Source: CAD feature listing. Evaluate the final solid. Frame: model axes, mm. Round coordinates to 2 decimals unless told otherwise and drop trailing zeros. Write each loop counter-clockwise with the first axis right and the second up, starting at its lowest first coordinate (ties: lowest second). Pieces come first, ordered by that corner, then holes. Notation, with made-up numbers: M -2,3.5 L 52,3.5 A27 cw 52,29.5 Z; hole C 23,36 d3. An arc over 180 degrees is marked long. Answer in a Markdown table with one row per item.
from build123d import *

# Parameters (mm, degrees)
F1_DEPTH = 3.5
F2_R     = 1.8
F3_DEPTH = 8
F4_R     = 1.8
F5_DEPTH = 8


with BuildPart() as f1:
    # F0 (on Top) → F1 (new body, symmetric)
    with BuildSketch(Plane.XY):
        with BuildLine():
            ThreePointArc((30, 1.5), (25.313708, 12.813708), (14, 17.5))
            Line((14, 17.5), (-14, 17.5))
            ThreePointArc((-14, 17.5), (-25.313708, 12.813708), (-30, 1.5))
            Line((-30, 1.5), (-30, -1.5))
            ThreePointArc((-30, -1.5), (-25.313708, -12.813708), (-14, -17.5))
            Line((-14, -17.5), (14, -17.5))
            ThreePointArc((14, -17.5), (25.313708, -12.813708), (30, -1.5))
            Line((30, -1.5), (30, 1.5))
        make_face()
    extrude(amount=F1_DEPTH, both=True)

    # F2 (on face) → F3 (cut)
    with BuildSketch(Plane.XY.offset(3.5)):
        with Locations((-22.338685, 0)):
            Circle(F2_R)
    extrude(amount=-F3_DEPTH, mode=Mode.SUBTRACT)

    # F4 (on face) → F5 (cut)
    with BuildSketch(Plane.XY.offset(3.5)):
        with Locations((21.90068, 0)):
            Circle(F4_R)
    extrude(amount=-F5_DEPTH, mode=Mode.SUBTRACT)


solid = f1.part
Q1. Pull-direction query (X, two-part tool) for faces 1 (the cylindrical face through (25.189, -12.937, 0.049)), 2 (the cylindrical face through (-25.437, -12.689, 0.049)), 3 (the cylindrical face through (23.618, 0.541, 0.049)), 4 (the flat face through (0, 17.5, 0)); classes: pulls with the +X half, pulls with the -X half, needs draft (parallel to the pull), parting line crosses it, or undercut.
Solutions:
| item | result |
|---|---|
| face 1 | pulls with the +X half |
| face 2 | pulls with the -X half |
| face 3 | undercut |
| face 4 | needs draft |
Q2. Section D-D (y = -5.5). Return loops of the section in (x, z).
Solutions:
| item | result |
|---|---|
| outline | M -29.49,-3.5 L 29.49,-3.5 L 29.49,3.5 L -29.49,3.5 Z |
Q3. Section A-A (y = 0). Return loops of the section in (x, z), and give its area (3 significant figures).
Solutions:
| item | result |
|---|---|
| outline | M -30,-3.5 L -24.14,-3.5 L -24.14,3.5 L -30,3.5 Z; M -20.54,-3.5 L 20.1,-3.5 L 20.1,3.5 L -20.54,3.5 Z; M 23.7,-3.5 L 30,-3.5 L 30,3.5 L 23.7,3.5 Z |
| area | 370 mm2 |
Q4. Contact query for flat-ended pins moving along their axis: pin 1 Ø1 at (y, z) = (-5.5, -1) entering from +X; pin 2 Ø4 at (y, z) = (10.5, -2.5) entering from +X; pin 3 Ø4.5 at (x, y) = (-22.34, 0) entering from -Z; pin 4 Ø1.5 at (x, z) = (-17, 2.5) entering from -Y. Output: stop coordinate, or through.
Solutions:
| item | result |
|---|---|
| pin 1 | stops at x = 29.61 |
| pin 2 | stops at x = 28.39 |
| pin 3 | stops at z = -3.5 |
| pin 4 | stops at y = -17.34 |
Q5. Section B-B (z = -0.25). Return loops of the section in (x, y).
Solutions:
| item | result |
|---|---|
| outline | M -30,-1.5 A16 ccw -14,-17.5 L 14,-17.5 A16 ccw 30,-1.5 L 30,1.5 A16 ccw 14,17.5 L -14,17.5 A16 ccw -30,1.5 Z; hole C -22.34,0 d3.6; hole C 21.9,0 d3.6 |
Q6. Material intervals for probe 1 along X at (y, z) = (1, -2.5); probe 2 along Y at (x, z) = (24, -0.5); probe 3 along Y at (x, z) = (-22, -2.5), sorted ascending.
Solutions:
| item | result |
|---|---|
| probe 1 | x = -30 to -23.84, -20.84 to 20.4, 23.4 to 30 |
| probe 2 | y = -13.99 to 13.99 |
| probe 3 | y = -15.36 to -1.77, 1.77 to 15.36 |
Q7. Section C-C (x = 17). Return loops of the section in (y, z).
Solutions:
| item | result |
|---|---|
| outline | M -17.22,-3.5 L 17.22,-3.5 L 17.22,3.5 L -17.22,3.5 Z |
